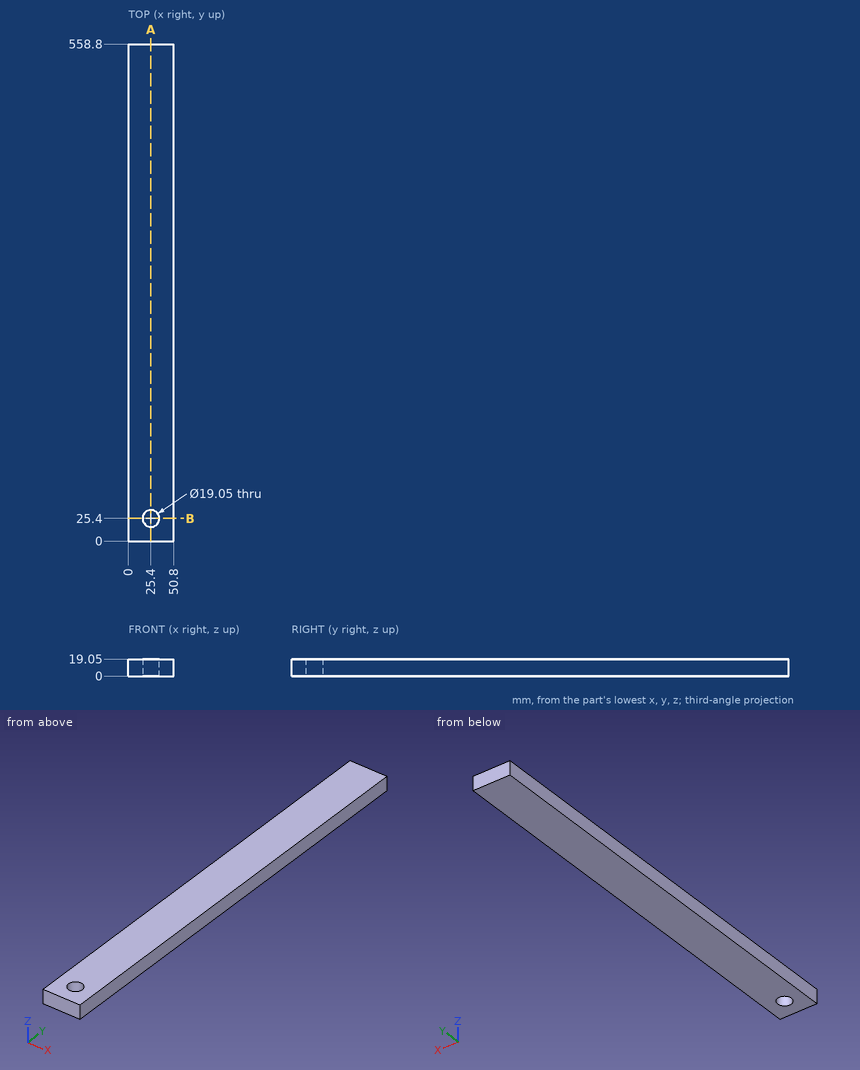
Geometry: see drawing. Coordinates: mm, zero at the bounding-box minimum. Give positions to 0.01 mm unless a question says otherwise; leave off trailing zeros. Loops run counter-clockwise (first coordinate to the right, second up) from the corner with the lowest first, then second, coordinate; pieces in that order, holes last. Notation, with made-up numbers: (-8, -25) -> (48, -25) arc R16 cw to (48, -4) -> close; hole circle Ø7 at (31, 17.5). An arc over 180 degrees is marked (long way). Answer as a JSON object with one key per item and string values. Group by question number.
Item 1: Cut plane A-A, the plane x = 25.4. Return the cut outline in (y, z) (3 decimals), and give its area (3 significant figures).
Item 2: Line query: probe 1 along Y at (x, z) = (25.4, 5) (3 decimals); probe 2 along Y at (x, z) = (30.5, 2.25). Output: solid intervals per line, ascending.
Item 3: Pin query (flat end, axial travel): P1, Ø3, axis at x = 33, y = 201.5, coming from the -Z side; P2, Ø11.5, axis at x = 25.4, y = 25.4, coming from the +Z side. Return the tip coordinate at first contact, or that it passes through.
Item 4: Cut plane B-B, the plane y = 25.4. Return the cut outline in (x, z) (3 decimals), and give its area (3 significant figures).
Checks:
{
 "1": {"outline": "(0, 0) -> (15.875, 0) -> (15.875, 19.05) -> (0, 19.05) -> close; (34.925, 0) -> (558.8, 0) -> (558.8, 19.05) -> (34.925, 19.05) -> close", "area": "10,300 mm²"},
 "2": {"probe 1": "y = 0 to 15.875, 34.925 to 558.8", "probe 2": "y = 0 to 17.36, 33.44 to 558.8"},
 "3": {"P1": "stops at z = 0", "P2": "passes through"},
 "4": {"outline": "(0, 0) -> (15.875, 0) -> (15.875, 19.05) -> (0, 19.05) -> close; (34.925, 0) -> (50.8, 0) -> (50.8, 19.05) -> (34.925, 19.05) -> close", "area": "605 mm²"}
}
